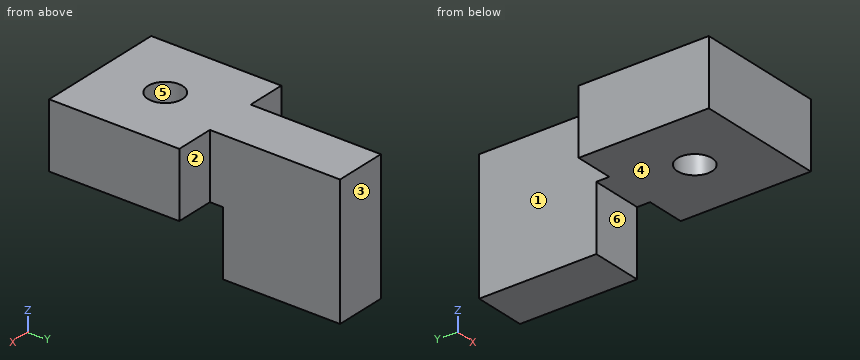
```python
from build123d import *

# Parameters (mm, degrees)
SKETCH1_W                  = 20
SKETCH1_H                  = 20
SKETCH1_W_2                = 8
BOSS_EXTRUDE1_DEPTH        = 10
F_4_0_209_DIAMETER_HOLE1_D = 5.3086
SKETCH1_3_W                = 8
SKETCH1_3_H                = 20
BOSS_EXTRUDE2_DEPTH        = 10
SKETCH4_W                  = 8
SKETCH4_H                  = 2
CUT_EXTRUDE1_DEPTH         = 10


with BuildPart() as part:
    # Sketch1 → Boss-Extrude1 (new body)
    with BuildSketch(Plane.XY):
        Rectangle(SKETCH1_W, SKETCH1_H)
        with Locations((0, 20)):
            Rectangle(SKETCH1_W_2, SKETCH1_H)
    extrude(amount=BOSS_EXTRUDE1_DEPTH)

    # #4 (0.209) Diameter Hole1 (through all)
    with Locations(Plane.XY.offset(10)):
        with Locations((0, 0)):
            Hole(F_4_0_209_DIAMETER_HOLE1_D / 2)

    # Sketch1<3> → Boss-Extrude2 (add)
    with BuildSketch(Plane.XY):
        with Locations((0, 20)):
            Rectangle(SKETCH1_3_W, SKETCH1_3_H)
    extrude(amount=-BOSS_EXTRUDE2_DEPTH)

    # Sketch4 → Cut-Extrude1 (cut)
    with BuildSketch(Plane(origin=(0, 0, -10), x_dir=(-1, 0, 0), z_dir=(0, 0, -1))):
        with Locations((0, 11)):
            Rectangle(SKETCH4_W, SKETCH4_H)
    extrude(amount=-CUT_EXTRUDE1_DEPTH, mode=Mode.SUBTRACT)


solid = part.part
```
Design review of the part built by this model. Coordinates are the model's own, in mm. Face numbers are marked on the shaded views. A direction names the side the tool comes from. Give positions to 0.01 mm unless a question says otherwise; leave off trailing zeros. Order: outer loops, then holes, each group sorted by start corner. A loop starts at its lowest first (then second) coordinate and runs counter-clockwise, first axis right, second up. Notation, with made-up numbers: M -33.75,-7.75 L -24.75,-7.75 A32 ccw -24.75,24.25 Z; hole C 24,89.5 d4. An arc over 180 degrees is marked long. One line per question, with ' | ' between items. Start each with the question number.
Q1. For L1, parallel to Y at x = 0, z = 2.5; L2, parallel to Z at x = -3.5, y = 2.5; L3, parallel to Y at x = 0.5, z = -1.5, list the stretches that pass through material, from the lowest coordinate up. Write a range as [from, to].
Q2. We need section B-B (y = 0). Write out the cut boundary in (x, z), plus the area to 3 significant figures.
Q3. Machinability: for the marked faces 1, 2 and 3, which of the approach directions +Z, -Z, +X, -X, +Y, -Y give a long, thin tool a straight path to every point of the face, cutting with its end or side? Answer none if there is none.
Q4. We need section D-D (y = -6.5). Write out the cut boundary in (x, z).
Q5. For pin 1 Ø3 at (y, z) = (15, 0.5) entering from +X; pin 2 Ø12 at (x, y) = (-3, 3.5) entering from -Z; pin 3 Ø6.5 at (x, z) = (-7.5, 5) entering from +Y, all flat-tipped, find the tip position at first contact; note any pin that passes through.
Q6. We need section A-A (x = 0). Write out the cut boundary in (y, z), plus the area to 3 significant figures.
Q7. We need section C-C (z = 6.5). Write out the cut boundary in (x, y), plus the area to 3 significant figures.
Q8. The part is to be moulded in two halves that separate along Y. For the marked faces 4, 5 and 6, say which applies: +Y half, -Y half, draft (parallel to the pull), parting line (faces both ways), or undercut.
Returned:
1) L1: [-10, -2.65], [2.65, 30] | L2: [0, 10] | L3: [12, 30]
2) outline: M -10,0 L -2.65,0 L -2.65,10 L -10,10 Z; M 2.65,0 L 10,0 L 10,10 L 2.65,10 Z | area: 147 mm2
3) face 1: +Z, -Z, -X, +Y | face 2: +Z, -Z, +X, +Y | face 3: +Z, -Z, +X, -X, +Y
4) outline: M -10,0 L 10,0 L 10,10 L -10,10 Z
5) pin 1: x = 4 | pin 2: z = 0 | pin 3: y = 10
6) outline: M -10,0 L -2.65,0 L -2.65,10 L -10,10 Z; M 2.65,0 L 12,0 L 12,-10 L 30,-10 L 30,10 L 2.65,10 Z | area: 527 mm2
7) outline: M -10,-10 L 10,-10 L 10,10 L 4,10 L 4,30 L -4,30 L -4,10 L -10,10 Z; hole C 0,0 d5.31 | area: 538 mm2
8) face 4: draft | face 5: undercut | face 6: -Y half
